Work out the finished part from the listing and answer in its coordinate system (mm). A direction names the side the tool comes from. Coordinates: 2 decimals unless noted, no trailing zeros. Write each loop counter-clockwise with the first axis right and the second up, starting at its lowest first coordinate (ties: lowest second). Pieces come first, ordered by that corner, then holes. Notation, with made-up numbers: M 47,-19 L 82,-19 A23 ccw 82,-10 Z; hole C 66,-18.75 d4. An arc over 180 degrees is marked long. Use CSV: the item, a comma, the result in double quotes.
from build123d import *

# Parameters (mm, degrees)
SKETCH1_R           = 11
BOSS_EXTRUDE1_DEPTH = 3
SKETCH2_R           = 8
BOSS_EXTRUDE2_DEPTH = 8
SKETCH3_R           = 11
BOSS_EXTRUDE3_DEPTH = 3
SKETCH4_R           = 1.55
CUT_EXTRUDE1_DEPTH  = 15
SKETCH5_R           = 0.75
CUT_EXTRUDE2_DEPTH  = 4


with BuildPart() as part:
    # Sketch1 → Boss-Extrude1 (new body)
    with BuildSketch(Plane.XY):
        Circle(SKETCH1_R)
    extrude(amount=BOSS_EXTRUDE1_DEPTH)

    # Sketch2 → Boss-Extrude2 (add)
    with BuildSketch(Plane.XY.offset(3)):
        Circle(SKETCH2_R)
    extrude(amount=BOSS_EXTRUDE2_DEPTH)

    # Sketch3 → Boss-Extrude3 (add)
    with BuildSketch(Plane.XY.offset(11)):
        Circle(SKETCH3_R)
    extrude(amount=BOSS_EXTRUDE3_DEPTH)

    # Sketch4 → Cut-Extrude1 (cut, through all)
    with BuildSketch(Plane.XY.offset(14)):
        Circle(SKETCH4_R)
    extrude(amount=-CUT_EXTRUDE1_DEPTH, mode=Mode.SUBTRACT)

    # Sketch5 → Cut-Extrude2 (cut, through all)
    with BuildSketch(Plane.XY.offset(3)):
        with Locations((0, 9)):
            Circle(SKETCH5_R)
    extrude(amount=-CUT_EXTRUDE2_DEPTH, mode=Mode.SUBTRACT)


solid = part.part
Item 1: The part is cut by section C-C (y = 9). Write down the section's boundary in (x, z), then the cut area to 3 significant figures.
Answer:
outline,"M -6.32,0 L -0.75,0 L -0.75,3 L -6.32,3 Z; M -6.32,11 L 6.32,11 L 6.32,14 L -6.32,14 Z; M 0.75,0 L 6.32,0 L 6.32,3 L 0.75,3 Z"
area,"71.4 mm2"
Item 2: The part is cut by section A-A (x = 0). Write down the section's boundary in (y, z).
Answer:
outline,"M -11,0 L -1.55,0 L -1.55,14 L -11,14 L -11,11 L -8,11 L -8,3 L -11,3 Z; M 1.55,0 L 8.25,0 L 8.25,3 L 8,3 L 8,11 L 11,11 L 11,14 L 1.55,14 Z; M 9.75,0 L 11,0 L 11,3 L 9.75,3 Z"
Item 3: For a pull along X with two mould halves and no side action, classify faces 1 (the face through (0.715, -1.375, 7.098)), 2 (the face through (-1.73, -7.81, 6.94)), 3 (the face through (0, -2, 0)) as released by +X, released by -X, zero draft, split by the parting line, or undercut.
Answer:
face 1,"undercut"
face 2,"split by the parting line"
face 3,"zero draft"
Item 4: A tool of negligible diameter and unlimited length cuts with its end or side. For faces 4 (the face through (0, -2, 14)), 5 (the face through (-0.098, 9.744, 1.521)), 6 (the face through (-6, -6, 3)), from which of +Z, -Z, +X, -X, +Y, -Y can it reach the whole face along a straight path? Write none if from no direction.
Answer:
face 4,"+Z, +X, -X, +Y, -Y"
face 5,"-Z"
face 6,"none"
Item 5: Consider probe 1 along Y at (x, z) = (0, 2.2); probe 2 along Y at (x, z) = (0, 10.25); probe 3 along Z at (x, y) = (6.5, -6). Determine where each line is inside the solid, lowest interval first.
Answer:
probe 1,"y = -11 to -1.55, 1.55 to 8.25, 9.75 to 11"
probe 2,"y = -8 to -1.55, 1.55 to 8"
probe 3,"z = 0 to 3, 11 to 14"
Item 6: Given pin 1 (6 mm diameter, centred on y = 5, z = 12.5, fed in from -X); pin 2 (2 mm diameter, centred on x = -3.5, z = 5, fed in from -Y); pin 3 (8 mm diameter, centred on x = 8.5, z = 5, fed in from +Y), each flat-ended and moving along its own axis, determine where each tip first touches the part or whether it passes through.
Answer:
pin 1,"stops at x = -10.82"
pin 2,"stops at y = -7.6"
pin 3,"stops at y = 9.78"
Item 7: The part is cut by section D-D (z = 12.5). Write down the section's boundary in (x, y), then the cut area to 3 significant figures.
Answer:
outline,"C 0,0 d22; hole C 0,0 d3.1"
area,"373 mm2"
Item 8: The part is cut by section B-B (y = 0). Write down the section's boundary in (x, z).
Answer:
outline,"M -11,0 L -1.55,0 L -1.55,14 L -11,14 L -11,11 L -8,11 L -8,3 L -11,3 Z; M 1.55,0 L 11,0 L 11,3 L 8,3 L 8,11 L 11,11 L 11,14 L 1.55,14 Z"
